```python
from build123d import *

# Parameters (mm, degrees)
SKETCH2_R           = 12.7
BOSS_EXTRUDE1_DEPTH = 44.45
BOSS_EXTRUDE3_DEPTH = 76.2
SKETCH5_3_W         = 22.225
SKETCH5_3_H         = 19.05
BOSS_EXTRUDE4_DEPTH = 95.25
CUT_EXTRUDE2_DEPTH  = 109.402793728
FILLET1_R           = 9.525


with BuildPart() as part:
    # Sketch2 → Boss-Extrude1 (new, symmetric)
    with BuildSketch(Plane.XY):
        with BuildLine():
            Line((-28.575, 0), (28.575, 0))
            Line((28.575, 0), (23.075738686, -9.525))
            Line((23.075738686, -9.525), (28.575, -9.525))
            Line((28.575, -9.525), (35.775738686, -9.525))
            Line((35.775738686, -9.525), (35.775738686, 19.449953455))
            ThreePointArc((35.775738686, 19.449953455), (0, 36.5125), (-35.775738686, 19.449953455))
            Line((-35.775738686, 19.449953455), (-35.775738686, -9.525))
            Line((-35.775738686, -9.525), (-28.575, -9.525))
            Line((-28.575, -9.525), (-23.075738686, -9.525))
            Line((-23.075738686, -9.525), (-28.575, 0))
        make_face()
        with Locations((0, 19.05)):
            Circle(SKETCH2_R, mode=Mode.SUBTRACT)
    extrude(amount=BOSS_EXTRUDE1_DEPTH, both=True)

    # Sketch5 → Boss-Extrude3 (add)
    with BuildSketch(Plane(origin=(0, 0, -44.45), x_dir=(-1, 0, 0), z_dir=(0, 0, -1))):
        with BuildLine():
            ThreePointArc((26.307142857, 28.255757549), (23.306989894, 31.663247782), (22.225, 36.072466007))
            Line((22.225, 36.072466007), (22.225, 76.2))
            Line((22.225, 76.2), (-22.225, 76.2))
            Line((-22.225, 76.2), (-22.225, 36.072466007))
            ThreePointArc((-22.225, 36.072466007), (-23.306989894, 31.663247782), (-26.307142857, 28.255757549))
            ThreePointArc((-26.307142857, 28.255757549), (0, 36.5125), (26.307142857, 28.255757549))
        make_face()
    extrude(amount=-BOSS_EXTRUDE3_DEPTH)

    # Sketch5_3 → Boss-Extrude4 (add)
    with BuildSketch(Plane(origin=(0, 0, -44.45), x_dir=(-1, 0, 0), z_dir=(0, 0, -1))):
        with Locations((-11.1125, 66.675)):
            Rectangle(SKETCH5_3_W, SKETCH5_3_H)
        with Locations((11.1125, 66.675)):
            Rectangle(SKETCH5_3_W, SKETCH5_3_H)
    extrude(amount=-BOSS_EXTRUDE4_DEPTH)

    # Sketch6 → Cut-Extrude2 (cut, through all)
    with BuildSketch(Plane(origin=(22.225, 0, 0), x_dir=(0, 0, -1), z_dir=(1, 0, 0))):
        with BuildLine():
            Line((44.45, 76.2), (-36.443114188, 76.2))
            ThreePointArc((-36.443114188, 76.2), (8.706401057, 65.616928498), (44.45, 36.072466007))
            Line((44.45, 36.072466007), (44.45, 76.2))
        make_face()
    extrude(amount=-CUT_EXTRUDE2_DEPTH, mode=Mode.SUBTRACT)

    # Fillet1
    fillet1_edges = [part.edges().sort_by_distance(p)[0] for p in [
        (0, 57.15, 31.75),
    ]]
    fillet(fillet1_edges, radius=FILLET1_R)


solid = part.part
```
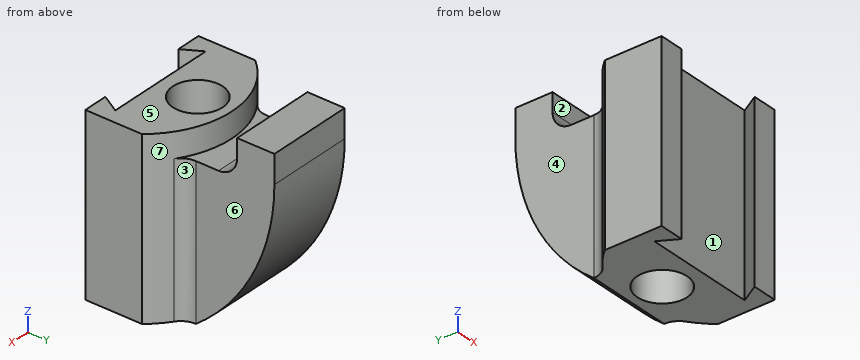
Could you check a few things on this model? Use its own coordinates, in mm. Face numbers are marked on the shaded views. A direction names the side the tool comes from. Coordinates: 2 decimals unless noted, no trailing zeros. Write each loop counter-clockwise with the first axis right and the second up, starting at its lowest first coordinate (ties: lowest second). Pieces come first, ordered by that corner, then holes. Notation, with made-up numbers: (52, -2) -> (108, -2) arc R15 ccw to (108, 3) -> close; hole circle Ø7 at (60.25, 41.25). An arc over 180 degrees is marked (long way). Return JSON: item names as keys, results as strings.
(1) We'd pull the mould along X, two halves only. Please class the marked faces 1, 2 and 3: +X half, -X half, draft (parallel to the pull), parting line (faces both ways), or undercut.
Numbers:
{"face 1": "undercut", "face 2": "draft", "face 3": "+X half"}
(2) I'm going to push flat-ended pins straight in: pin 1 (8 mm diameter, centred on x = -20, z = 10.5, fed in from +Y); pin 2 (5 mm diameter, centred on y = 28.5, z = -34.5, fed in from -X); pin 3 (5 mm diameter, centred on x = -4, y = 42.5, fed in from -Z). Where does each tip first touch, or does it pass through?
Numbers:
{"pin 1": "stops at y = 73.8", "pin 2": "stops at x = -29.28", "pin 3": "stops at z = -41.31"}
(3) Which directions (+Z, -Z, +X, -X, +Y, -Y) give clear straight access to the entire face, cutting with the end or side of a thin tool? Please do the marked faces 4, 5, 6 and 7.
Numbers:
{"face 4": "+Z, -Z, -X, +Y", "face 5": "+Z, +X, -X, -Y", "face 6": "+Z, -Z, +X, +Y", "face 7": "+Z"}
(4) Imagine slicing it at C-C, the plane y = 34.5. Please give me the cut outline in (x, z).
Numbers:
{"outline": "(-22.36, -44.45) -> (22.36, -44.45) -> (22.36, 31.75) -> (13.46, 31.75) -> (13.46, 44.45) -> (-13.46, 44.45) -> (-13.46, 31.75) -> (-22.36, 31.75) -> close"}
(5) I need wall thicknesses on L1, parallel to X at y = 19, z = -7; L2, parallel to Z at x = -13.5, y = 26; L3, parallel to X at y = 61, z = 39 (3 decimals). Which ranges of each line are inside material? Lowest first, please.
Numbers:
{"L1": "x = -35.78 to -12.7, 12.7 to 35.78", "L2": "z = -44.45 to 44.45", "L3": "x = -22.225 to 22.225"}
